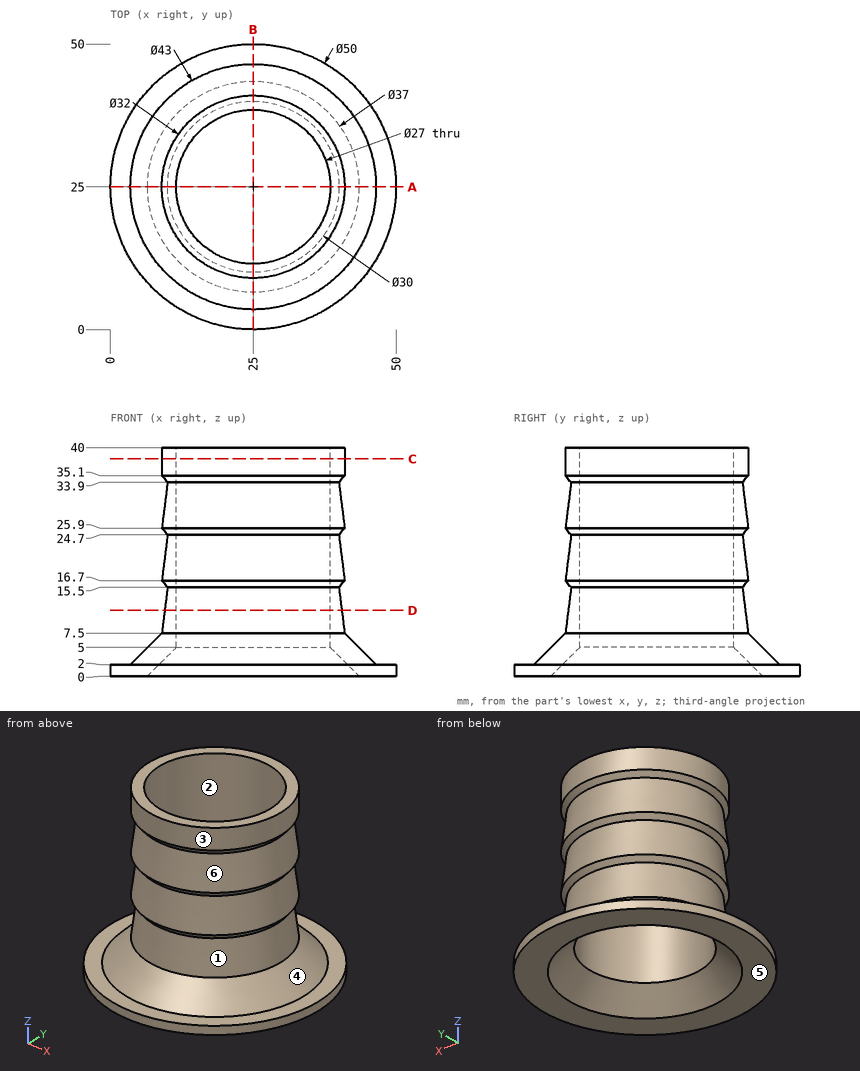
Geometry: see drawing. Coordinates: mm, zero at the bounding-box minimum. A direction names the side the tool comes from. Give positions to 0.01 mm unless a question says otherwise; leave off trailing zeros. Order: outer loops, then holes, each group sorted by start corner. A loop starts at its lowest first (then second) coordinate and runs counter-clockwise, first axis right, second up. Notation, with made-up numbers: M 15.25,35.25 L 52.25,35.25 A36 ccw 52.25,73.25 Z; hole C 2,11.5 d8. An arc over 180 degrees is marked long. Answer as a JSON object with one key per item and string values.
1. Reachability of the marked faces 1, 2 and 3 from +Z, -Z, +X, -X, +Y, -Y: full face, straight path, thin tool, end or side. Return the list, or none.
Result sheet:
{"face 1": "none", "face 2": "+Z, -Z", "face 3": "+Z"}
2. Cut plane D-D, the plane z = 11.5. Output: boundary loops of the cut face in (x, y).
Result sheet:
{"outline": "C 25,25 d31; hole C 25,25 d27"}
3. First-contact query: P1, Ø5, axis at x = 5.5, y = 29, coming from the +Z side; P2, Ø6, axis at x = 17, z = 28.5, coming from the -Y side; P3, Ø12, axis at x = 19, z = 33, coming from the +Y side. Flat tips, straight axial feed; report the tip coordinate or a pass-through.
Result sheet:
{"P1": "z = 6.09", "P2": "y = 10.07", "P3": "y = 41"}
4. Cut plane A-A, the plane y = 25. Output: boundary loops of the cut face in (x, z), and give its area (3 significant figures).
Result sheet:
{"outline": "M 0,0 L 6.5,0 L 11.5,5 L 11.5,40 L 9,40 L 9,35.1 L 10,33.9 L 9,25.9 L 10,24.7 L 9,16.7 L 10,15.5 L 9,7.5 L 3.5,2 L 0,2 Z; M 38.5,5 L 43.5,0 L 50,0 L 50,2 L 46.5,2 L 41,7.5 L 40,15.5 L 41,16.7 L 40,24.7 L 41,25.9 L 40,33.9 L 41,35.1 L 41,40 L 38.5,40 Z", "area": "214 mm²"}
5. Pull-direction query (Z, two-part tool) for the marked faces 4, 5 and 6; classes: +Z half, -Z half, draft (parallel to the pull), parting line (faces both ways), or undercut.
Result sheet:
{"face 4": "+Z half", "face 5": "-Z half", "face 6": "undercut"}
6. Ray query, line 1 (X direction, y = 16, z = 8); line 2 (Y direction, x = 31.5, z = 26.5); line 3 (Y direction, x = 25.5, z = 21). Return the intervals inside material, ascending. Write a range as [from, to].
Result sheet:
{"line 1": "[11.85, 14.94], [35.06, 38.15]", "line 2": "[10.46, 13.17], [36.83, 39.54]", "line 3": "[9.55, 11.51], [38.49, 40.45]"}
7. Cut plane C-C, the plane z = 38. Output: boundary loops of the cut face in (x, y), and give its area (3 significant figures).
Result sheet:
{"outline": "C 25,25 d32; hole C 25,25 d27", "area": "232 mm²"}
